The model under review builds one solid part; all positions refer to its coordinate system, in mm. Face numbers are marked on the shaded views. A direction names the side the tool comes from. Round coordinates to 2 decimals unless told otherwise and drop trailing zeros. Write each loop counter-clockwise with the first axis right and the second up, starting at its lowest first coordinate (ties: lowest second). Pieces come first, ordered by that corner, then holes. Notation, with made-up numbers: (43, 26) - (63, 26) arc R21 cw to (63, 47) - close; hole circle Ø5 at (43, 52.5). An arc over 180 degrees is marked (long way). Write each question's results on one line, items separated by ' | '.
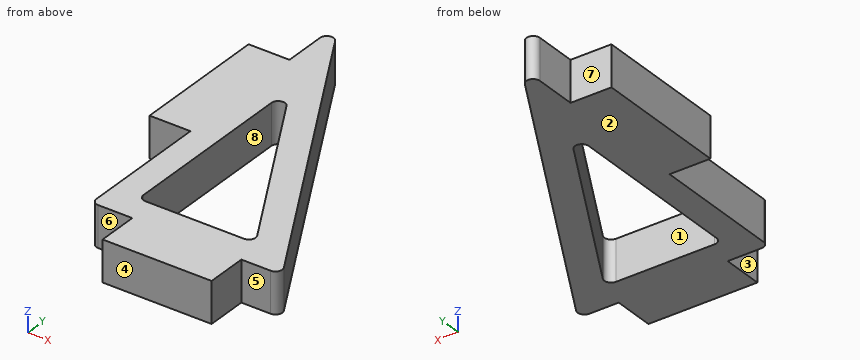
```python
from build123d import *

# Parameters (mm, degrees)
EXTRUDE_2_DEPTH     = 3
CUT_EXTRUDE_1_DEPTH = 28.412321808


with BuildPart() as part:
    # 草图1 → 凸台-拉伸2 (new body)
    with BuildSketch(Plane.XY):
        with BuildLine():
            Line((0.5, 0), (3, 0))
            Line((3, 0), (3, -3))
            Line((3, -3), (11, -3))
            Line((11, -3), (11, 0))
            Line((11, 0), (13.146938049, 0))
            ThreePointArc((13.146938049, 0), (13.578302652, 0.247166895), (13.583191057, 0.744301684))
            Line((13.583191057, 0.744301684), (0.936253008, 23.328119629))
            ThreePointArc((0.936253008, 23.328119629), (0.373759167, 23.567618783), (0, 23.083817944))
            Line((0, 23.083817944), (0, 20))
            Line((0, 20), (-3, 20))
            Line((-3, 20), (-3, 10))
            Line((-3, 10), (0, 10))
            Line((0, 10), (0, 0.5))
            ThreePointArc((0, 0.5), (0.146446609, 0.146446609), (0.5, 0))
        make_face()
    extrude(amount=EXTRUDE_2_DEPTH)

    # 草图2 → 切除-拉伸1 (cut, through all)
    with BuildSketch(Plane.XY.offset(3)):
        with BuildLine():
            Line((2, 15.419089721), (2, 2.5))
            ThreePointArc((2, 2.5), (2.146446609, 2.146446609), (2.5, 2))
            Line((2.5, 2), (9.734690244, 2))
            ThreePointArc((9.734690244, 2), (10.166054847, 2.247166895), (10.170943252, 2.744301684))
            Line((10.170943252, 2.744301684), (2.936253008, 15.663391405))
            ThreePointArc((2.936253008, 15.663391405), (2.373759167, 15.90289056), (2, 15.419089721))
        make_face()
    extrude(amount=-CUT_EXTRUDE_1_DEPTH, mode=Mode.SUBTRACT)


solid = part.part
```
Q1. We need section A-A (z = 2.5). State the section outline as (x, y) points, plus the area to 3 significant figures.
Evaluation:
outline: (-3, 10) - (0, 10) - (0, 0.5) arc R0.5 ccw to (0.5, 0) - (3, 0) - (3, -3) - (11, -3) - (11, 0) - (13.15, 0) arc R0.5 ccw to (13.58, 0.74) - (0.94, 23.33) arc R0.5 ccw to (0, 23.08) - (0, 20) - (-3, 20) - close; hole (2, 2.5) arc R0.5 ccw to (2.5, 2) - (9.73, 2) arc R0.5 ccw to (10.17, 2.74) - (2.94, 15.66) arc R0.5 ccw to (2, 15.42) - close | area: 163 mm^2
Q2. We need section D-D (x = -2). State the section outline as (y, z) points.
Evaluation:
outline: (10, 0) - (20, 0) - (20, 3) - (10, 3) - close
Q3. For probe 1 along X at (y, z) = (-0.25, 0.4); probe 2 along X at (y, z) = (15.75, 1.65); probe 3 along Y at (x, z) = (8, 1.15), list the stretches that pass through material, from the lowest coordinate up.
Evaluation:
probe 1: x = 3 to 11 | probe 2: x = -3 to 2.13, 2.87 to 5.18 | probe 3: y = -3 to 2, 6.62 to 10.71
Q4. The part is to be moulded in two halves that separate along X. For the marked faces 1, 2 and 3, say which applies: released by +X, released by -X, zero draft, split by the parting line, or undercut.
Evaluation:
face 1: undercut | face 2: zero draft | face 3: released by -X
Q5. Insertion check: P1, Ø5, axis at x = 8, y = 13.5, coming from the -Z side; P2, Ø1, axis at y = 16.5, z = 1, coming from the +X side; P3, Ø1.5, axis at x = -1.5, z = 1, coming from the +Y side; P4, Ø0.9, axis at y = 3.5, z = 1, coming from the -X side. Each pin has a flat end and moves straight along its axis. Give the tip position at first contact, or say it passes through.
Evaluation:
P1: stops at z = 0 | P2: stops at x = 5.04 | P3: stops at y = 20 | P4: stops at x = 0
Q6. We need section B-B (x = 9.25). State the section outline as (y, z) points.
Evaluation:
outline: (-3, 0) - (2, 0) - (2, 3) - (-3, 3) - close; (4.39, 0) - (8.48, 0) - (8.48, 3) - (4.39, 3) - close
Q7. We need section C-C (y = 19.5). State the section outline as (x, z) points, plus the area to 3 significant figures.
Evaluation:
outline: (-3, 0) - (3.08, 0) - (3.08, 3) - (-3, 3) - close | area: 18.2 mm^2
Q8. Tool access review of the marked faces 4, 5, 6, 7 and 8: name each direction out of +Z, -Z, +X, -X, +Y, -Y from which nothing blocks a thin tool from reaching the whole face with its end or side.
Evaluation:
face 4: +Z, -Z, +X, -X, -Y | face 5: +Z, -Z, +X, -Y | face 6: +Z, -Z, -X, -Y | face 7: +Z, -Z, -X, +Y | face 8: +Z, -Z
